Geometry check sheet. Reference: the model listing, model coordinates, mm. A direction names the side the tool comes from. Coordinates: 2 decimals unless noted, no trailing zeros. One line per question, with ' | ' between items.
```python
from build123d import *

# Parameters (mm, degrees)
EXTRUDE_1_DEPTH     = 39
SKETCH_7_R          = 1.65
CUT_EXTRUDE_1_DEPTH = 10
SKETCH_11_R         = 1.5
CUT_EXTRUDE_2_DEPTH = 10
SKETCH_12_W         = 29.009042243
SKETCH_12_H         = 10
CUT_EXTRUDE_3_DEPTH = 40
SKETCH_14_R         = 3
CUT_EXTRUDE_4_DEPTH = 0.7
SKETCH_17_W         = 22.396032982
SKETCH_17_H         = 19.376343142
CUT_EXTRUDE_5_DEPTH = 48
SKETCH_18_W         = 48.955276493
SKETCH_18_H         = 0.5
SKETCH_18_W_2       = 40.156862745
CUT_EXTRUDE_6_DEPTH = 150


with BuildPart() as part:
    # 草图1 → 凸台-拉伸1 (new body)
    with BuildSketch(Plane.XY):
        Polygon((18.538024786, -87.708726548), (18.538024786, -75.708726548), (-3.150193841, 47.291273452), (-1.119340617, 47.291273452), (20.538024786, -75.533749221), (20.538024786, -87.708726548), align=None)
    extrude(amount=EXTRUDE_1_DEPTH)

    # 草图7 → 切除-拉伸1 (cut)
    with BuildSketch(Plane(origin=(7.001695694, 1.234587862, 0), x_dir=(0, 0, -1), z_dir=(0.9848077530122079, 0.17364817766693164, 0))):
        with Locations(Location((-30, -19.232815796, 0), (0, 0, 90))):
            Circle(SKETCH_7_R)
        with Locations(Location((-9, -19.232815796, 0), (0, 0, 90))):
            Circle(SKETCH_7_R)
        with Locations(Location((-30, -12.732815796, 0), (0, 0, 90))):
            Circle(SKETCH_7_R)
        with Locations(Location((-9, -12.732815796, 0), (0, 0, 90))):
            Circle(SKETCH_7_R)
        with Locations(Location((-9, -25.732815796, 0), (0, 0, 90))):
            Circle(SKETCH_7_R)
        with Locations(Location((-30, -25.732815796, 0), (0, 0, 90))):
            Circle(SKETCH_7_R)
    extrude(amount=-CUT_EXTRUDE_1_DEPTH, mode=Mode.SUBTRACT)

    # 草图11 → 切除-拉伸2 (cut)
    with BuildSketch(Plane(origin=(5.032080188, 0.887291506, 0), x_dir=(0, 0, 1), z_dir=(-0.9848077530122079, -0.1736481776669316, 0))):
        with Locations(Location((5, 12.119838165, 0), (0, 0, 270))):
            Circle(SKETCH_11_R)
        with Locations(Location((34, 12.119838165, 0), (0, 0, 270))):
            Circle(SKETCH_11_R)
    extrude(amount=-CUT_EXTRUDE_2_DEPTH, mode=Mode.SUBTRACT)

    # 草图12 → 切除-拉伸3 (cut)
    with BuildSketch(Plane.XY.offset(39)):
        with Locations((0.338832517, 47.079233545)):
            Rectangle(SKETCH_12_W, SKETCH_12_H)
    extrude(amount=-CUT_EXTRUDE_3_DEPTH, mode=Mode.SUBTRACT)

    # 草图14 → 切除-拉伸4 (cut)
    with BuildSketch(Plane(origin=(7.001695694, 1.234587862, 0), x_dir=(0, 0, -1), z_dir=(0.9848077530122078, 0.17364817766693164, 0))):
        with Locations(Location((-34, 12.119838165, 0), (0, 0, 90))):
            Circle(SKETCH_14_R)
        with Locations(Location((-5, 12.119838165, 0), (0, 0, 90))):
            Circle(SKETCH_14_R)
        with Locations(Location((-30, -19.232815796, 0), (0, 0, 90))):
            Circle(SKETCH_14_R)
        with Locations(Location((-9, -19.232815796, 0), (0, 0, 90))):
            Circle(SKETCH_14_R)
        with Locations(Location((-30, -12.732815796, 0), (0, 0, 90))):
            Circle(SKETCH_14_R)
        with Locations(Location((-9, -12.732815796, 0), (0, 0, 90))):
            Circle(SKETCH_14_R)
        with Locations(Location((-30, -25.732815796, 0), (0, 0, 90))):
            Circle(SKETCH_14_R)
        with Locations(Location((-9, -25.732815796, 0), (0, 0, 90))):
            Circle(SKETCH_14_R)
    extrude(amount=-CUT_EXTRUDE_4_DEPTH, mode=Mode.SUBTRACT)

    # 草图17 → 切除-拉伸5 (cut)
    with BuildSketch(Plane(origin=(0, 0, 0), x_dir=(-1, 0, 0), z_dir=(0, 0, -1))):
        with Locations((2.347013145, 39.90800246)):
            Rectangle(SKETCH_17_W, SKETCH_17_H)
    extrude(amount=-CUT_EXTRUDE_5_DEPTH, mode=Mode.SUBTRACT)

    # 草图18 → 切除-拉伸6 (cut)
    with BuildSketch(Plane(origin=(0, 30.219830889, 0), x_dir=(1, 0, 0), z_dir=(0, 1, 0))):
        with Locations((4.107783916, -0.25)):
            Rectangle(SKETCH_18_W, SKETCH_18_H)
        with Locations((8.50699079, -38.75)):
            Rectangle(SKETCH_18_W_2, SKETCH_18_H)
    extrude(amount=-CUT_EXTRUDE_6_DEPTH, mode=Mode.SUBTRACT)


solid = part.part
```
(1) Material ranges on line 1 (X direction, y = -79, z = 26); line 2 (X direction, y = 4, z = 15.5), recorded low to high.
Answers below:
line 1: x = 18.54 to 20.54 | line 2: x = 4.48 to 6.51
(2) Cross-section at A-A (y = 13). Count the separate pieces of the cut face and the enclosed holes in it, plus the area to 3 significant figures.
Answers below:
separate pieces: 3 | enclosed holes: 0 | area: 60.7 mm²
(3) Draft check along Z on faces 3 (the face through (12, -33, 38.5)), 4 (the face through (8.59, -9.78, 32.53)), 5 (the face through (11.084, -21.917, 19.234)). Enter one of: pulls with the +Z half, pulls with the -Z half, needs draft (parallel to the pull), parting line crosses it, or undercut.
Answers below:
face 3: pulls with the +Z half | face 4: undercut | face 5: needs draft
(4) Depth check by flat-ended pin: P1, Ø10, axis at x = 6.5, z = 22, coming from the +Y side; P2, Ø9.5, axis at y = -80, z = 23, coming from the -X side; P3, Ø5, axis at y = -71.5, z = 14, coming from the -X side. Enter the tip coordinate at first touch or a pass-through.
Answers below:
P1: stops at y = 30.22 | P2: stops at x = 18.46 | P3: stops at x = 17.36
(5) Tool access check on faces 1 (the face through (4.67, 12.47, 2.07)), 2 (the face through (18.538, -82, 19)). Record the directions out of +Z, -Z, +X, -X, +Y, -Y that give a thin tool (end or side, any length) a straight path to the whole face; none if there is none.
Answers below:
face 1: none | face 2: +Z, -Z, -X, -Y
